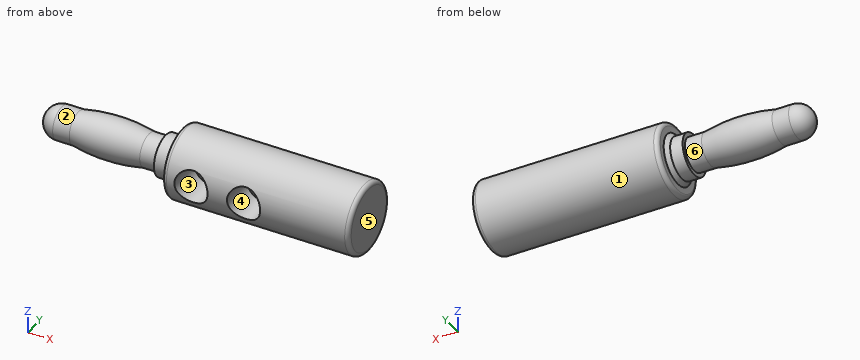
from build123d import *

# Parameters (mm, degrees)
CHAMFER1_SIZE      = 0.5
FILLET1_R          = 0.5
SKETCH3_R          = 2
CUT_EXTRUDE1_DEPTH = 25.4


with BuildPart() as part:
    # Sketch1 → Revolve1 (revolve)
    with BuildSketch(Plane.XY):
        with BuildLine():
            Line((0, 0), (-39, 0))
            ThreePointArc((-39, 0), (-38.414213562, 1.414213562), (-37, 2))
            Line((-37, 2), (-35, 2))
            ThreePointArc((-35, 2), (-30.75, 2.432654399), (-26.5, 2))
            Line((-26.5, 2), (-24.5, 2))
            Line((-24.5, 2), (-24.5, 2.5))
            Line((-24.5, 2.5), (-22.5, 2.5))
            Line((-22.5, 2.5), (-22.5, 4.25))
            Line((-22.5, 4.25), (0, 4.25))
            Line((0, 4.25), (0, 0))
        make_face()
    revolve(axis=Axis((-39, 0, 0), (-1, 0, 0)))

    # Chamfer1
    chamfer1_edges = [part.edges().sort_by_distance(p)[0] for p in [
        (-22.5, -2.5, 0),
    ]]
    chamfer(chamfer1_edges, length=CHAMFER1_SIZE)

    # Fillet1
    fillet1_edges = [part.edges().sort_by_distance(p)[0] for p in [
        (0, -4.25, 0),
        (-22.5, -4.25, 0),
    ]]
    fillet(fillet1_edges, radius=FILLET1_R)

    # Sketch3 → Cut-Extrude1 (cut)
    with BuildSketch(Plane(origin=(0, 0, 0), x_dir=(1, 0, 0), z_dir=(0, 1, 0))):
        with Locations(Location((-19.05, 0, 0), (0, 0, 270))):
            Circle(SKETCH3_R)
        with Locations(Location((-12.7, 0, 0), (0, 0, 270))):
            Circle(SKETCH3_R)
    extrude(amount=-CUT_EXTRUDE1_DEPTH, mode=Mode.SUBTRACT)


solid = part.part
Check sheet for the modelled part. Datum: model origin and axes. Units: mm. Face numbers are marked on the shaded views. A direction names the side the tool comes from. Coordinates: 2 decimals unless noted, no trailing zeros. Loops run counter-clockwise (first coordinate to the right, second up) from the corner with the lowest first, then second, coordinate; pieces in that order, holes last. Notation, with made-up numbers: (-26, 88.25) -> (23, 88.25) arc R14 ccw to (23, 94.25) -> close; hole circle Ø11 at (39.5, -25.75). An arc over 180 degrees is marked (long way). Answer in a Markdown table with one row per item.
1. Release check for a two-part mould opening along Z. For the marked faces 4, 5 and 6 record: released by +Z, released by -Z, zero draft, split by the parting line, or undercut.
Check values:
| item | result |
|---|---|
| face 4 | undercut |
| face 5 | zero draft |
| face 6 | split by the parting line |
2. Sectioned sample at C-C, the plane x = -10. Record the boundary of the cut face in (y, z), then the cut area to 3 significant figures.
Check values:
| item | result |
|---|---|
| outline | circle Ø8.5 at (0, 0) |
| area | 56.7 mm2 |
3. Material ranges on line 1 along X through (y, z) = (-3.3, 0); line 2 along X through (y, z) = (-1.7, 0); line 3 along Y through (x, z) = (-5.5, -3.75), recorded low to high. Write a range as [from, to].
Check values:
| item | result |
|---|---|
| line 1 | x = [-22.5, -21.05], [-17.05, -14.7], [-10.7, 0] |
| line 2 | x = [-38.05, -21.05], [-17.05, -14.7], [-10.7, 0] |
| line 3 | y = [-2, 2] |
4. Go/stop test with flat-tipped pins: pin 1 (4 mm diameter, centred on x = -26, y = -3, fed in from +Z); pin 2 (1 mm diameter, centred on x = -22, z = 2.5, fed in from -Y); pin 3 (1.2 mm diameter, centred on x = -19.5, z = -0.5, fed in from -Y). Record where each tip stops, or that it passes through.
Check values:
| item | result |
|---|---|
| pin 1 | stops at z = 1.85 |
| pin 2 | stops at y = -3.75 |
| pin 3 | stops at y = 0 |
5. Access from +Z, -Z, +X, -X, +Y, -Y to the whole of each face (thin tool, end or side, straight path). Record for the marked faces 1, 2 and 3.
Check values:
| item | result |
|---|---|
| face 1 | +X, -X |
| face 2 | -X |
| face 3 | -Y |
6. Sectioned sample at A-A, the plane x = -19.05. Record the boundary of the cut face in (y, z).
Check values:
| item | result |
|---|---|
| outline | (-3.75, -2) arc R4.25 ccw (long way) to (-3.75, 2) -> (0, 2) -> (0, -2) -> close |
7. Sectioned sample at B-B, the plane y = -1.5. Give the number of separate pieces and of enclosed holes in the cut face, then the cut area to 3 significant figures.
Check values:
| item | result |
|---|---|
| separate pieces | 1 |
| enclosed holes | 2 |
| area | 205 mm2 |
